Check sheet for the modelled part. Datum: model origin and axes. Units: mm. Face numbers are marked on the shaded views. Coordinates: 2 decimals unless noted, no trailing zeros. Loops run counter-clockwise (first coordinate to the right, second up) from the corner with the lowest first, then second, coordinate; pieces in that order, holes last. Notation, with made-up numbers: (69, 89.5) -> (127, 89.5) arc R15 ccw to (127, 110.5) -> close; hole circle Ø7 at (-14.75, 84). An arc over 180 degrees is marked (long way). Use one line per item in the form item = value.
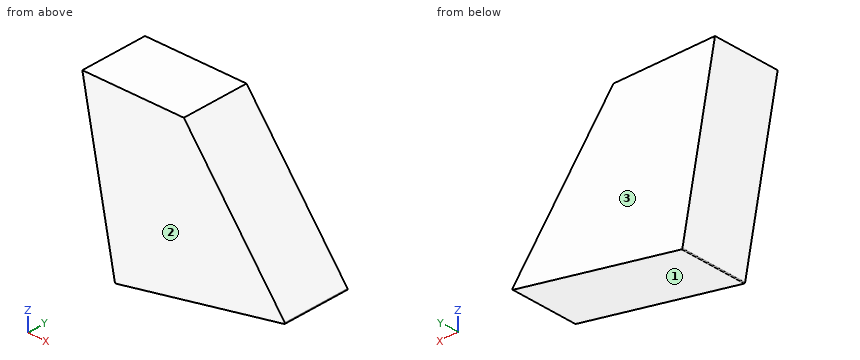
from build123d import *

# Parameters (mm, degrees)
F1_DEPTH = 508


with BuildPart() as f1:
    # F0 (on Front) → F1 (new body)
    with BuildSketch(Plane.XZ):
        with BuildLine():
            ThreePointArc((-508.468338, -841.325435), (-505.78588, -845.378186), (-501.023368, -846.34713))
            Line((-501.023368, -846.34713), (763.527564, -600.543329))
            ThreePointArc((763.527564, -600.543329), (768.244163, -596.585633), (767.387262, -590.488471))
            Line((767.387262, -590.488471), (9.197902, 415.662793))
            Line((9.197902, 415.662793), (-752.802098, 415.662793))
            Line((-752.802098, 415.662793), (-508.468338, -841.325435))
        make_face()
    extrude(amount=F1_DEPTH)


solid = f1.part
(1) Section check B-B, the plane z = -375. Record the boundary of the cut face in (x, y).
Established:
outline = (-599.11, -508) -> (605.01, -508) -> (605.01, 0) -> (-599.11, 0) -> close
(2) Scan lines: line 1 along X through (y, z) = (-399.5, -237); line 2 along Z through (x, y) = (-485, -71.5); line 3 along X through (y, z) = (-143.5, 36.5). Record each from-to range of solid material in increasing order.
Established:
line_1 = -625.94 to 501.01
line_2 = -843.23 to 415.66
line_3 = -679.1 to 294.92
(3) Mould release check, pull along Y, two halves, no side actions. Record for the marked faces 1, 2 and 3: +Y half, -Y half, draft (parallel to the pull), parting line (faces both ways), or undercut.
Established:
face_1 = draft
face_2 = -Y half
face_3 = +Y half
(4) Section check C-C, the plane x = 656. Record the boundary of the cut face in (y, z).
Established:
outline = (-508, -621.44) -> (0, -621.44) -> (0, -442.67) -> (-508, -442.67) -> close
(5) Go/stop test with flat-tipped pins: P1, Ø1.5, axis at x = 84.5, y = -103, coming from the -Z side; P2, Ø3, axis at y = -148.5, z = 259.5, coming from the -X side; P3, Ø1, axis at y = -300, z = -193, coming from the +X side (3 decimals). Record where each tip stops, or that it passes through.
Established:
P1 = -732.68
P2 = -722.74
P3 = 468.235
(6) Section check A-A, the plane y = -188. Record the boundary of the cut face in (x, z) (3 decimals).
Established:
outline = (-752.802, 415.663) -> (-508.468, -841.325) arc R6.35 ccw to (-501.023, -846.347) -> (763.528, -600.543) arc R6.35 ccw to (767.387, -590.488) -> (9.198, 415.663) -> close
